Geometry check sheet. Reference: the model listing, model coordinates, mm. A direction names the side the tool comes from. Coordinates: 2 decimals unless noted, no trailing zeros. Loops run counter-clockwise (first coordinate to the right, second up) from the corner with the lowest first, then second, coordinate; pieces in that order, holes last. Notation, with made-up numbers: (29.25, 40) - (82.25, 40) arc R24 cw to (82.25, 75) - close; hole circle Ø2 at (73.5, -24.5). An arc over 180 degrees is marked (long way). Write each question's results on one line, items separated by ' | '. Start each with the question number.
(1) Access from +Z, -Z, +X, -X, +Y, -Y to the whole of each face (thin tool, end or side, straight path). Record for faces 5 (the face through (-15, 0, -31)), 6 (the face through (-47.02, 253.5, -28.02)).
(2) Material ranges on probe 1 along X at (y, z) = (169.5, 12.5); probe 2 along Z at (x, y) = (-33.5, 77) (3 decimals); probe 3 along X at (y, z) = (254, 29.5), recorded low to high.
(3) Sectioned sample at B-B (y = 40). Enter the section's corners in (x, z) (3 decimals).
(4) Sectioned sample at C-C (x = 10). Enter the section's corners in (y, z) (3 decimals), plus the area to 3 significant figures.
(5) Sectioned sample at A-A (z = -7). Enter the section's corners in (x, y).
(6) Mould release check, pull along X, two halves, no side actions. Record for faces 1 (the face through (-51.25, 254, 0)), 2 (the face through (49.5, 254, 0)), 3 (the face through (47.02, 253.5, 28.02)), 4 (the face through (51.25, 254, 0)): pulls with the +X half, pulls with the -X half, needs draft (parallel to the pull), parting line crosses it, or undercut.
from build123d import *

# Parameters (mm, degrees)
F1_DEPTH = 300


# Not quite as in the source:
# - a pattern or mirror of a feature is missing from the dataset's text; its kind, count and spacing are read off the source's solid


with BuildPart() as f1:
    # F0 (on Front) → F1 (new body)
    with BuildSketch(Plane.XZ):
        with BuildLine():
            ThreePointArc((51.25, 22.125), (48.3210678119, 29.1960678119), (41.25, 32.125))
            Line((41.25, 32.125), (-41.25, 32.125))
            ThreePointArc((-41.25, 32.125), (-48.3210678119, 29.1960678119), (-51.25, 22.125))
            Line((-51.25, 22.125), (-51.25, -22.125))
            ThreePointArc((-51.25, -22.125), (-48.3210678119, -29.1960678119), (-41.25, -32.125))
            Line((-41.25, -32.125), (41.25, -32.125))
            ThreePointArc((41.25, -32.125), (48.3210678119, -29.1960678119), (51.25, -22.125))
            Line((51.25, -22.125), (51.25, 22.125))
        make_face()
        with BuildLine():
            Line((-49.5, -22.125), (-49.5, 22.125))
            ThreePointArc((-49.5, 22.125), (-47.0836309448, 27.9586309448), (-41.25, 30.375))
            Line((-41.25, 30.375), (41.25, 30.375))
            ThreePointArc((41.25, 30.375), (47.0836309448, 27.9586309448), (49.5, 22.125))
            Line((49.5, 22.125), (49.5, -22.125))
            ThreePointArc((49.5, -22.125), (47.0836309448, -27.9586309448), (41.25, -30.375))
            Line((41.25, -30.375), (-41.25, -30.375))
            ThreePointArc((-41.25, -30.375), (-47.0836309448, -27.9586309448), (-49.5, -22.125))
        make_face(mode=Mode.SUBTRACT)
    extrude(amount=-F1_DEPTH)

    # F1_copies: F1 across plane


with BuildPart() as f1_1:
    add(f1.part)
    add(f1.part.mirror(Plane.ZX.offset(250)))


solid = f1_1.part
Outcome:
1) face 5: +Z, -Z, +X, -X, -Y | face 6: +Y, -Y
2) probe 1: x = -51.25 to -49.5, 49.5 to 51.25 | probe 2: z = -32.125 to -30.375, 30.375 to 32.125 | probe 3: x = -48 to -44.95, 44.95 to 48
3) outline: (-51.25, -22.125) arc R10 ccw to (-41.25, -32.125) - (41.25, -32.125) arc R10 ccw to (51.25, -22.125) - (51.25, 22.125) arc R10 ccw to (41.25, 32.125) - (-41.25, 32.125) arc R10 ccw to (-51.25, 22.125) - close; hole (-49.5, -22.125) arc R8.25 ccw to (-41.25, -30.375) - (41.25, -30.375) arc R8.25 ccw to (49.5, -22.125) - (49.5, 22.125) arc R8.25 ccw to (41.25, 30.375) - (-41.25, 30.375) arc R8.25 ccw to (-49.5, 22.125) - close
4) outline: (0, -32.125) - (500, -32.125) - (500, -30.375) - (0, -30.375) - close; (0, 30.375) - (500, 30.375) - (500, 32.125) - (0, 32.125) - close | area: 1,750 mm2
5) outline: (-51.25, 0) - (-49.5, 0) - (-49.5, 500) - (-51.25, 500) - close; (49.5, 0) - (51.25, 0) - (51.25, 500) - (49.5, 500) - close
6) face 1: pulls with the -X half | face 2: undercut | face 3: undercut | face 4: pulls with the +X half
